Read the model definition and answer for the solid it produces. Units are mm, in the model's axes. Coordinates: 2 decimals unless noted, no trailing zeros. Order: outer loops, then holes, each group sorted by start corner. A loop starts at its lowest first (then second) coordinate and runs counter-clockwise, first axis right, second up. Notation, with made-up numbers: M 39.25,51.25 L 49.25,51.25 A19 cw 49.25,66.25 Z; hole C 36,21 d10. An arc over 180 degrees is marked long. Use a Markdown table: item, result. Add a question column.
1) Find the intervals of material crossed by probe 1 along X at (y, z) = (-4, -33.5); probe 2 along Z at (x, y) = (-394, -7); probe 3 along Z at (x, y) = (-151, -3.5), in increasing order. Write a range as [from, to].
2) Find section A-A on x = -112. Write down the section's boundary in (y, z).
3) Each of these flat-tipped pins is pushed along its axis until it touches: pin 1 Ø15.5 at (x, z) = (190.5, 74.5) entering from -Y; pin 2 Ø4 at (x, y) = (-264, 8.5) entering from -Z; pin 3 Ø12 at (y, z) = (6, 51.5) entering from +X; pin 4 Ø12 at (x, y) = (275, 5.5) entering from -Z. Where does it stop, or does it pass through?
4) Find section B-B on z = 49. Write down the section's boundary in (x, y), plus the area to 3 significant figures.
from build123d import *

# Parameters (mm, degrees)
F1_W     = 40
F1_H     = 33
F3_DEPTH = 600
F2_W     = 80
F2_H     = 100
F4_DEPTH = 25


with BuildPart() as f3:
    # F1 (on Right) → F3 (new body, symmetric)
    with BuildSketch(Plane.YZ):
        Polygon((20, 33), (20, 63), (17, 66), (12, 66), (12, 80), (4, 80), (4, 66), (-4, 66), (-4, 80), (-12, 80), (-12, 66), (-17, 66), (-20, 63), (-20, 33), align=None)
        with Locations((0, 16.5)):
            Rectangle(F1_W, F1_H)
        with Locations((0, -16.5)):
            Rectangle(F1_W, F1_H)
        Polygon((20, -63), (20, -33), (-20, -33), (-20, -63), (-17, -66), (-12, -66), (-12, -52), (-4, -52), (-4, -66), (4, -66), (4, -52), (12, -52), (12, -66), (17, -66), align=None)
    extrude(amount=F3_DEPTH, both=True)

    # F2 (on Front) → F4 (cut, symmetric)
    with BuildSketch(Plane.XZ):
        with Locations((600, 83)):
            Rectangle(F2_W, F2_H)
        with Locations((600, -83)):
            Rectangle(F2_W, F2_H)
    extrude(amount=F4_DEPTH, both=True, mode=Mode.SUBTRACT)


solid = f3.part
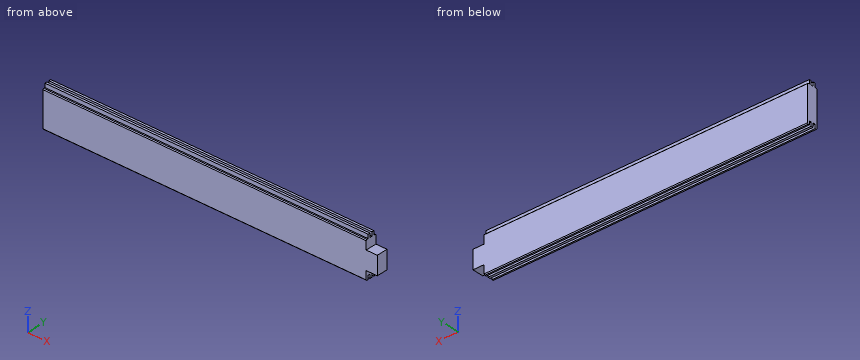
Check result:
| question | item | result |
|---|---|---|
| 1 | probe 1 | x = [-600, 560] |
| 1 | probe 2 | z = [-52, 80] |
| 1 | probe 3 | z = [-66, 66] |
| 2 | outline | M -20,-63 L -17,-66 L -12,-66 L -12,-52 L -4,-52 L -4,-66 L 4,-66 L 4,-52 L 12,-52 L 12,-66 L 17,-66 L 20,-63 L 20,63 L 17,66 L 12,66 L 12,80 L 4,80 L 4,66 L -4,66 L -4,80 L -12,80 L -12,66 L -17,66 L -20,63 Z |
| 3 | pin 1 | stops at y = -12 |
| 3 | pin 2 | stops at z = -52 |
| 3 | pin 3 | stops at x = 560 |
| 3 | pin 4 | stops at z = -66 |
| 4 | outline | M -600,-20 L 560,-20 L 560,20 L -600,20 Z |
| 4 | area | 46,400 mm2 |
